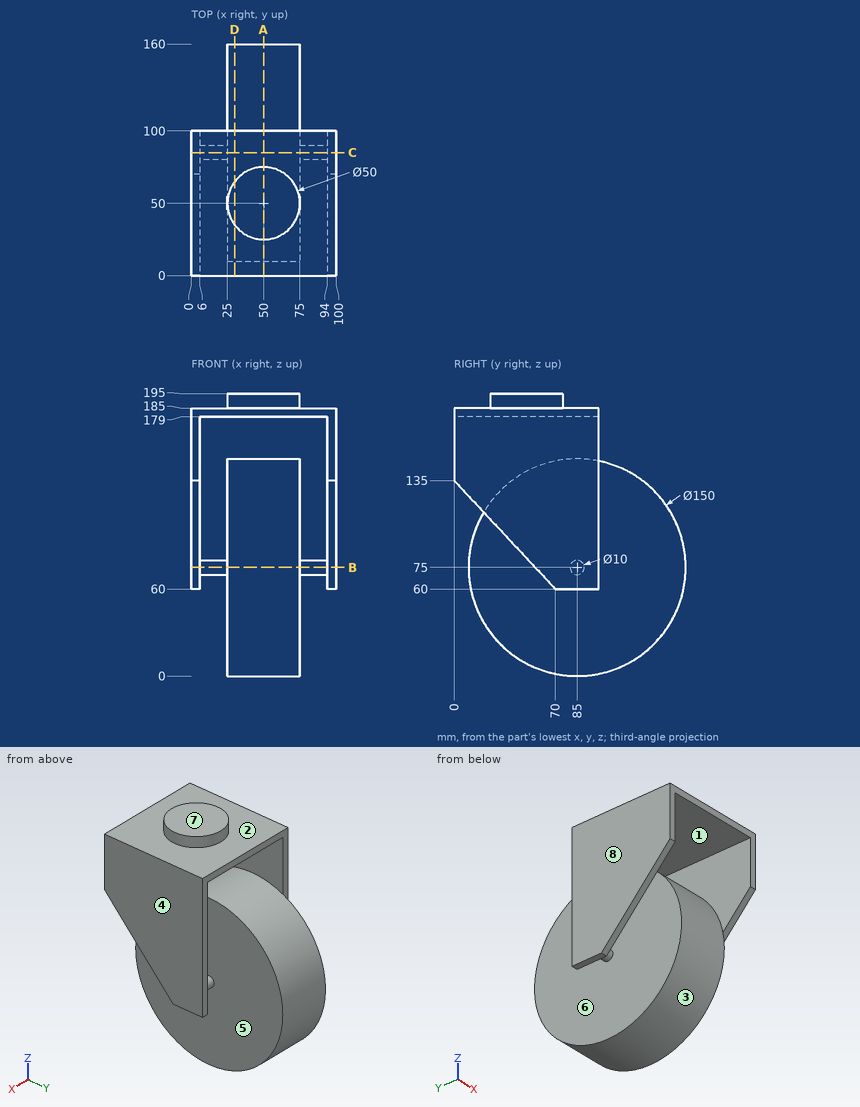
Check sheet for the drawn part. Datum: minimum x, y, z corner. Units: mm. A direction names the side the tool comes from. Round coordinates to 2 decimals unless told otherwise and drop trailing zeros. Order: outer loops, then holes, each group sorted by start corner. A loop starts at its lowest first (then second) coordinate and runs counter-clockwise, first axis right, second up.
1) Scan lines: line 1 (X direction, y = 44.5, z = 129.5); line 2 (X direction, y = 36.5, z = 154); line 3 (Z direction, x = 42, y = 38). Record each from-to range of solid material in increasing order.
2) Section check C-C (y = 85). Record the boundary of the cut face in (x, z), and give its area (3 significant figures).
3) Section check A-A (x = 50). Record the boundary of the cut face in (y, z).
4) Go/stop test with flat-tipped pins: pin 1 Ø3 at (x, y) = (30, 27.5) entering from -Z; pin 2 Ø1 at (y, z) = (113.5, 25) entering from +X; pin 3 Ø1 at (x, y) = (13, 24.5) entering from -Z. Record where each tip stops, or that it passes through.
5) Section check B-B (z = 75). Record the boundary of the cut face in (x, y), and give its area (3 significant figures).
6) Tool access check on the marked faces 1, 2, 3 and 4. Record the directions out of +Z, -Z, +X, -X, +Y, -Y that give a thin tool (end or side, any length) a straight path to the whole face; none if there is none.
7) Section check D-D (x = 30). Record the boundary of the cut face in (y, z), and give its area (3 significant figures).
8) Mould release check, pull along X, two halves, no side actions. Record for the marked faces 5, 6, 7 and 8: +X half, -X half, draft (parallel to the pull), parting line (faces both ways), or undercut.
Result:
1. line 1: x = 0 to 6, 25 to 75, 94 to 100
1. line 2: x = 0 to 6, 94 to 100
1. line 3: z = 16.55 to 133.45, 179 to 195
2. outline: (0, 60) - (6, 60) - (6, 70) - (25, 70) - (25, 0) - (75, 0) - (75, 70) - (94, 70) - (94, 60) - (100, 60) - (100, 185) - (0, 185) - close; hole (6, 80) - (25, 80) - (25, 150) - (75, 150) - (75, 80) - (94, 80) - (94, 179) - (6, 179) - close
2. area: 9,910 mm2
3. outline: (0, 179) - (100, 179) - (100, 185) - (75, 185) - (75, 195) - (25, 195) - (25, 185) - (0, 185) - close; circle Ø150 at (85, 75)
4. pin 1: stops at z = 25.11
4. pin 2: stops at x = 75
4. pin 3: stops at z = 179
5. outline: (0, 56) - (6, 56) - (6, 80) - (25, 80) - (25, 10) - (75, 10) - (75, 80) - (94, 80) - (94, 56) - (100, 56) - (100, 100) - (94, 100) - (94, 90) - (75, 90) - (75, 160) - (25, 160) - (25, 90) - (6, 90) - (6, 100) - (0, 100) - close
5. area: 8,410 mm2
6. face 1: +Y, -Y
6. face 2: +Z
6. face 3: none
6. face 4: +Z, -Z, +X, +Y, -Y
7. outline: (0, 179) - (100, 179) - (100, 185) - (65, 185) - (65, 195) - (35, 195) - (35, 185) - (0, 185) - close; circle Ø150 at (85, 75)
7. area: 18,600 mm2
8. face 5: undercut
8. face 6: undercut
8. face 7: draft
8. face 8: -X half
